Read the model definition and answer for the solid it produces. Units are mm, in the model's axes. A direction names the side the tool comes from. Round coordinates to 2 decimals unless told otherwise and drop trailing zeros. Order: outer loops, then holes, each group sorted by start corner. A loop starts at its lowest first (then second) coordinate and runs counter-clockwise, first axis right, second up. Notation, with made-up numbers: (27.5, -3.75) -> (37.5, -3.75) arc R24 ccw to (37.5, 27.25) -> close; hole circle Ø8 at (71, 86.5). An arc over 180 degrees is marked (long way). One line per item, written item: value. Start each with the question number.
1. Flat-ended cylindrical pins translate along their axes: pin 1 Ø3.5 at (x, y) = (-1.5, -7.5) entering from -Z; pin 2 Ø1.5 at (x, z) = (-4.5, -0.5) entering from -Y; pin 3 Ø2.5 at (x, y) = (0.5, -6.5) entering from +Z. Find the tip coordinate at first contact, or state that the pin passes through.
2. For faces 4 (the face through (-3.905, 0.493, -0.867)), 5 (the face through (0, -7, 2)), 6 (the face through (1.5, -2.7, -2)), determine the directions among +Z, -Z, +X, -X, +Y, -Y from which every point of the face is accessible in a straight line to the end or side of a thin tool.
3. Section A-A (y = -0.25) is taken. Give the vertices of the cut face in (x, z), then the cut area to 3 significant figures.
4. The mould has two halves that part along Y. Classify faces 1 (the face through (6, -6, 0)), 2 (the face through (0, 1, 0)), 3 (the face through (2, 0, 2)): released by +Y, released by -Y, zero draft, split by the parting line, or undercut.
5. Consider line 1 (Z direction, x = -1.75, y = -6.5); line 2 (Y direction, x = 1.5, z = -3); line 3 (Z direction, x = 2, y = -2.5). Determine where each line is inside the solid, lowest interval first.
from build123d import *

# Parameters (mm, degrees)
SKETCH1_R               = 4
BOSS_EXTRUDE1_DEPTH     = 1
SKETCH2_R               = 2.5
BOSS_EXTRUDE2_DEPTH     = 5.4
SKETCH3_W               = 12
SKETCH3_H               = 4
BOSS_EXTRUDE3_DEPTH     = 3
CUT_EXTRUDE1_DEPTH      = 12.939849245
CUT_EXTRUDE1_DEPTH_BACK = 12.939849245
CUT_EXTRUDE2_DEPTH      = 12.070682133
CUT_EXTRUDE2_DEPTH_BACK = 12.070682133


with BuildPart() as part:
    # Sketch1 → Boss-Extrude1 (new body)
    with BuildSketch(Plane(origin=(0, 0, 0), x_dir=(1, 0, 0), z_dir=(0, 1, 0))):
        with Locations(Location((0, 0, 0), (0, 0, 270))):
            Circle(SKETCH1_R)
    extrude(amount=BOSS_EXTRUDE1_DEPTH)

    # Sketch2 → Boss-Extrude2 (add)
    with BuildSketch(Plane(origin=(0, 0, 0), x_dir=(-1, 0, 0), z_dir=(0, -1, 0))):
        with Locations(Location((0, 0, 0), (0, 0, 270))):
            Circle(SKETCH2_R)
    extrude(amount=BOSS_EXTRUDE2_DEPTH)

    # Sketch3 → Boss-Extrude3 (add)
    with BuildSketch(Plane.XZ.offset(5.4)):
        Rectangle(SKETCH3_W, SKETCH3_H)
    extrude(amount=BOSS_EXTRUDE3_DEPTH)

    # Sketch4 → Cut-Extrude1 (cut, two sides: drawn at the far end of the back side and taken through both)
    with BuildSketch(Plane(origin=(0, 0, -2), x_dir=(-1, 0, 0), z_dir=(0, 0, -1)).offset(-CUT_EXTRUDE1_DEPTH_BACK)):
        with BuildLine():
            Line((-6, -6.9), (-6.927802535, -6.9))
            Line((-6.927802535, -6.9), (-6.927802535, -9.790233254))
            Line((-6.927802535, -9.790233254), (7.497210963, -9.790233254))
            Line((7.497210963, -9.790233254), (7.497210963, -6.84173926))
            Line((7.497210963, -6.84173926), (6, -6.9))
            add(Edge.make_bspline(
                [(6, -6.9), (0, -9.9), (-6, -6.9)],
                knots=[0, 0, 0, 1, 1, 1], degree=2))
        make_face()
    extrude(amount=CUT_EXTRUDE1_DEPTH + CUT_EXTRUDE1_DEPTH_BACK, mode=Mode.SUBTRACT)

    # Sketch5 → Cut-Extrude2 (cut, two sides: drawn at the far end of the back side and taken through both)
    with BuildSketch(Plane(origin=(0, 0, 0), x_dir=(0, 0, -1), z_dir=(1, 0, 0)).offset(-CUT_EXTRUDE2_DEPTH_BACK)):
        with BuildLine():
            Line((2.5, -1.11050973), (3.286969074, -1.11050973))
            Line((3.286969074, -1.11050973), (3.286969074, -6.28949027))
            Line((3.286969074, -6.28949027), (2, -5.4))
            add(Edge.make_bspline(
                [(2.5, -1.11050973), (2.094671437, -3.238964164), (2, -5.4)],
                knots=[0, 0, 0, 1, 1, 1], degree=2))
        make_face()
        with BuildLine():
            Line((-3.286969074, -6.28949027), (-2, -5.4))
            add(Edge.make_bspline(
                [(-2.5, -1.11050973), (-2.094671437, -3.238964164), (-2, -5.4)],
                knots=[0, 0, 0, 1, 1, 1], degree=2))
            Line((-2.5, -1.11050973), (-3.286969074, -1.11050973))
            Line((-3.286969074, -1.11050973), (-3.286969074, -6.28949027))
        make_face()
    extrude(amount=CUT_EXTRUDE2_DEPTH + CUT_EXTRUDE2_DEPTH_BACK, mode=Mode.SUBTRACT)


solid = part.part
Answer:
1. pin 1: z = -2
1. pin 2: y = -7.81
1. pin 3: z = 2.01
2. face 4: +Y
2. face 5: +Z, +X, -X, -Y
2. face 6: none
3. outline: circle Ø5 at (0, 0)
3. area: 19.6 mm^2
4. face 1: zero draft
4. face 2: released by +Y
4. face 3: undercut
5. line 1: -2 to 2
5. line 2: 0 to 1
5. line 3: -1.5 to 1.5
